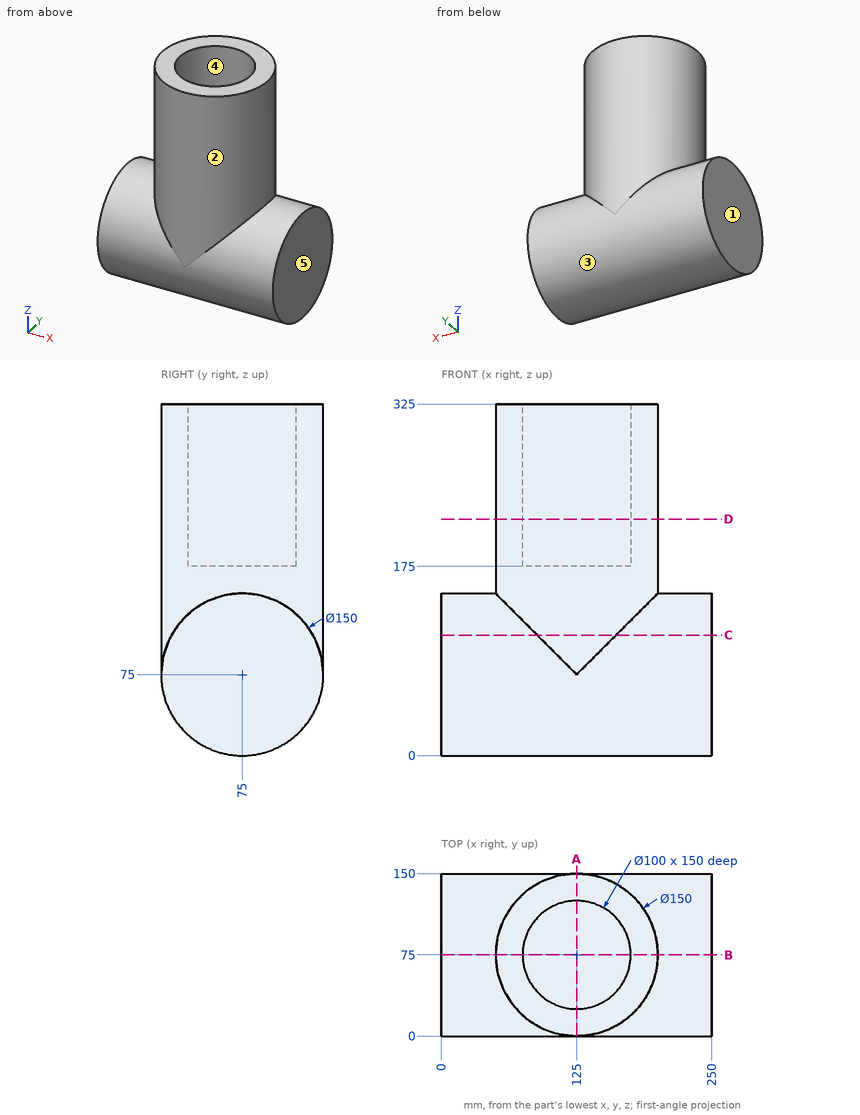
The figure shows three views and two pictorial views of one solid part (mm, origin at its lowest corner). Answer the questions. A direction names the side the tool comes from. Give positions to 0.01 mm unless a question says otherwise; leave off trailing zeros. Order: outer loops, then holes, each group sorted by start corner. A loop starts at its lowest first (then second) coordinate and runs counter-clockwise, first axis right, second up. Notation, with made-up numbers: (-18.5, 3.5) -> (23.5, 3.5) arc R9 ccw to (23.5, 9.5) -> close; hole circle Ø3 at (82.25, 17). An arc over 180 degrees is marked (long way). Answer as a JSON object with one key per item and string values. Group by question number.
Item 1: The part is cut by section D-D on z = 218.5. Write down the section's boundary in (x, y).
Item 2: The part is cut by section A-A on x = 125. Write down the section's boundary in (y, z), and give its area (3 significant figures).
Item 3: The part is cut by section B-B on y = 75. Write down the section's boundary in (x, z), and give its area (4 significant figures).
Item 4: A tool of negligible diameter and unlimited length cuts with its end or side. For the marked faces 1 and 2, from which of +Z, -Z, +X, -X, +Y, -Y can it reach the whole face along a straight path? Write none if from no direction.
Item 5: The part is cut by section C-C on z = 111.5. Write down the section's boundary in (x, y), and give its area (3 significant figures).
Item 6: Consider L1, parallel to Y at x = 139, z = 265.5; L2, parallel to Y at x = 139.5, z = 206; L3, parallel to Z at x = 154, y = 142. Determine where each line is inside the solid, lowest interval first. Write a range as from..to.
Item 7: Flat-ended cylindrical pins translate along their axes: pin 1 (5 mm diameter, centred on x = 153.5, z = 51.5, fed in from +Y); pin 2 (6 mm diameter, centred on x = 71.5, y = 77.5, fed in from -Z); pin 3 (3 mm diameter, centred on y = 96, z = 247, fed in from -X); pin 4 (10 mm diameter, centred on x = 39, y = 58, fed in from -Z). Find the tip coordinate at first contact, or state that the pin passes through.
Item 8: Determine the mould class of the marked faces 3, 4 and 5 for opening direction Y: pulls with the +Y half, pulls with the -Y half, needs draft (parallel to the pull), parting line crosses it, or undercut.
Result set:
{
 "1": {"outline": "circle Ø150 at (125, 75); hole circle Ø100 at (125, 75)"},
 "2": {"outline": "(0, 75) arc R75 ccw to (150, 75) -> (150, 325) -> (125, 325) -> (125, 175) -> (25, 175) -> (25, 325) -> (0, 325) -> close", "area": "31,300 mm²"},
 "3": {"outline": "(0, 0) -> (250, 0) -> (250, 150) -> (200, 150) -> (200, 325) -> (175, 325) -> (175, 175) -> (75, 175) -> (75, 325) -> (50, 325) -> (50, 150) -> (0, 150) -> close", "area": "48,750 mm²"},
 "4": {"face 1": "+Z, -Z, -X, +Y, -Y", "face 2": "+Z"},
 "5": {"outline": "(0, 9.48) -> (88.5, 9.48) arc R75 ccw to (161.5, 9.48) -> (250, 9.48) -> (250, 140.52) -> (161.5, 140.52) arc R75 ccw to (88.5, 140.52) -> (0, 140.52) -> close", "area": "33,700 mm²"},
 "6": {"L1": "1.32..27, 123..148.68", "L2": "1.42..27.15, 122.85..148.58", "L3": "41.3..325"},
 "7": {"pin 1": "y = 147", "pin 2": "z = 0", "pin 3": "x = 52.58", "pin 4": "z = 0.97"},
 "8": {"face 3": "parting line crosses it", "face 4": "undercut", "face 5": "needs draft"}
}
